Model file for the job. Use its own axes, mm. Face numbers are marked on the shaded views. A direction names the side the tool comes from. Round coordinates to 2 decimals unless told otherwise and drop trailing zeros. Loops run counter-clockwise (first coordinate to the right, second up) from the corner with the lowest first, then second, coordinate; pieces in that order, holes last. Notation, with made-up numbers: M 55.25,74 L 62.25,74 A7 ccw 62.25,82 Z; hole C 78.5,67 d3. An arc over 180 degrees is marked long. Use a Markdown table: item, result. Add a question column.
Item 1: Saw through at B-B on y = 5.75. Write the cut outline in (x, z), then the cut area to 3 significant figures.
Item 2: Saw through at A-A on y = 1. Write the cut outline in (x, z), then the cut area to 3 significant figures.
Item 3: Tool access for the marked faces 1 and 2: list every direction of +Z, -Z, +X, -X, +Y, -Y with a clear straight run to the whole face (end or side of a thin tool).
Item 4: Pin check, flat tips, straight feed: P1, Ø1.4, axis at y = 1.5, z = -0.5, coming from the -X side; P2, Ø2, axis at x = -1.5, z = -1.5, coming from the +Y side; P3, Ø0.8, axis at x = 0.5, y = 1, coming from the +Z side; P4, Ø1.5, axis at y = 7.5, z = 0.5, coming from the -X side. Stop position of each tip, or through.
Item 5: Saw through at C-C on y = 7.5. Write the cut outline in (x, z), then the cut area to 3 significant figures.
Item 6: Wall check: L1, parallel to Y at x = 0.8, z = 0.3; L2, parallel to X at y = 2.75, z = -1.15; L3, parallel to X at y = 7, z = 0.35. Give the ranges that are in metal, low to high. Write a range as from..to.
Item 7: Two-plate mould, pull along X, no slides. Class the marked faces 3, 4 and 5: +X half, -X half, draft (parallel to the pull), parting line (faces both ways), or undercut.
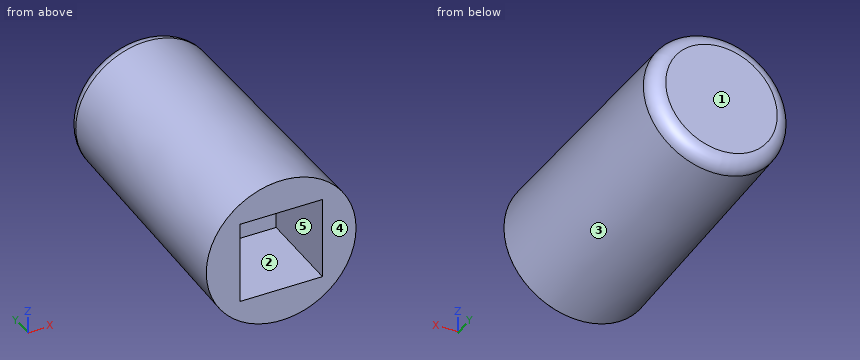
Autodesk Inventor part; units mm, degrees
ref_plane "YZ Plane" through (0, 0, 0) normal (1, 0, 0) x (0, 1, 0)
ref_plane "XZ Plane" through (0, 0, 0) normal (0, 1, 0) x (-1, 0, 0)
ref_plane "XY Plane" through (0, 0, 0) normal (0, 0, 1) x (1, 0, 0)
sketch "Sketch1" plane through (0, 0, 0) normal (0, 1, 0) x (-1, 0, 0)
  circle A0 centre (0, 0) radius 2.54
  dimension "d0" = 5.08
extrude "Extrusion1" add sketch "Sketch1" along normal blind 9.09
chamfer "Chamfer1" distance 9.09 angle 1 1 edges at (2.54, 9.09, 0) measured on face at (-2.5071, 3.03, -0.4074)
fillet "Fillet1" radius 0.5 1 edges at (2.3818, 9.09, 0)
sketch "Sketch2" plane through (0, 0, 0) normal (0, -1, 0) x (1, 0, 0)
  line L0 (1.4, -1.4) -> (-1.4, -1.4)
  line L1 (-1.4, -1.4) -> (-1.4, 1.4)
  line L2 (-1.4, 1.4) -> (1.4, 1.4)
  line L3 (1.4, 1.4) -> (1.4, -1.4)
  point P0 (0, 0)
  dimension "d7" = 2.8
  dimension "d8" = 1.4
  dimension "d9" = 2.8
  dimension "d10" = 1.4
extrude "Extrusion2" cut sketch "Sketch2" against normal blind 2.95
properties part number "1RBLK_TactileCap"
Entries:
| question | item | result |
|---|---|---|
| 1 | outline | C 0,0 d4.88 |
| 1 | area | 18.7 mm2 |
| 2 | outline | C 0,0 d5.05; hole M -1.4,-1.4 L 1.4,-1.4 L 1.4,1.4 L -1.4,1.4 Z |
| 2 | area | 12.2 mm2 |
| 3 | face 1 | +Z, -Z, +X, -X, +Y |
| 3 | face 2 | -Y |
| 4 | P1 | x = -2.52 |
| 4 | P2 | y = 9.09 |
| 4 | P3 | z = 2.52 |
| 4 | P4 | x = -2.42 |
| 5 | outline | C 0,0 d4.82 |
| 5 | area | 18.2 mm2 |
| 6 | L1 | 2.95..9.09 |
| 6 | L2 | -2.21..-1.4, 1.4..2.21 |
| 6 | L3 | -2.39..2.39 |
| 7 | face 3 | parting line |
| 7 | face 4 | draft |
| 7 | face 5 | undercut |
